from build123d import *

# Parameters (mm, degrees)
SKETCH1_W               = 260
SKETCH1_H               = 60
BOSS_EXTRUDE1_DEPTH     = 5
SKETCH2_W               = 5
SKETCH2_H               = 30
SKETCH2_W_2             = 220
SKETCH2_H_2             = 3
CUT_EXTRUDE1_DEPTH      = 140.73546436
CUT_EXTRUDE2_DEPTH      = 140.73546436
CUT_EXTRUDE2_DEPTH_BACK = 140.73546436
SKETCH3_R               = 1.45
SKETCH3_R_2             = 1.95


with BuildPart() as part:
    # Sketch1 → Boss-Extrude1 (new body)
    with BuildSketch(Plane.XY):
        with Locations((0, 21)):
            Rectangle(SKETCH1_W, SKETCH1_H)
    extrude(amount=BOSS_EXTRUDE1_DEPTH)

    # Sketch2 → Cut-Extrude1 (cut, through all)
    with BuildSketch(Plane.XY.offset(5)):
        with Locations((-127.5, 21)):
            Rectangle(SKETCH2_W, SKETCH2_H)
        with Locations((0, 49.5)):
            Rectangle(SKETCH2_W_2, SKETCH2_H_2)
        with Locations((127.5, 21)):
            Rectangle(SKETCH2_W, SKETCH2_H)
        with BuildLine():
            Line((108, -2), (-108, -2))
            ThreePointArc((-108, -2), (-103.050252532, -4.050252532), (-101, -9))
            Line((-101, -9), (101, -9))
            ThreePointArc((101, -9), (103.050252532, -4.050252532), (108, -2))
        make_face()
        with BuildLine():
            Line((108, -9), (115, -9))
            ThreePointArc((115, -9), (112.949747468, -4.050252532), (108, -2))
            Line((108, -2), (108, -9))
        make_face()
        with BuildLine():
            Line((108, -9), (108, -2))
            ThreePointArc((108, -2), (103.050252532, -4.050252532), (101, -9))
            Line((101, -9), (108, -9))
        make_face()
        with BuildLine():
            ThreePointArc((-108, -2), (-112.949747468, -4.050252532), (-115, -9))
            Line((-115, -9), (-108, -9))
            Line((-108, -9), (-108, -2))
        make_face()
        with BuildLine():
            ThreePointArc((-101, -9), (-103.050252532, -4.050252532), (-108, -2))
            Line((-108, -2), (-108, -9))
            Line((-108, -9), (-101, -9))
        make_face()
    extrude(amount=-CUT_EXTRUDE1_DEPTH, mode=Mode.SUBTRACT)

    # Sketch3 → Cut-Extrude2 (cut, two sides: drawn at the far end of the back side and taken through both)
    with BuildSketch(Plane.XY.offset(5).offset(-CUT_EXTRUDE2_DEPTH_BACK)):
        Polygon((-96.45, 43.2), (-96.45, 40), (-93.55, 40), (-93.55, 43.2), (-92.325, 43.2), (-92.325, 45.5), (-93.55, 45.5), (-93.55, 48), (-96.45, 48), (-96.45, 45.5), (-97.675, 45.5), (-97.675, 43.2), align=None)
        Polygon((97.675, 43.2), (97.675, 45.5), (96.45, 45.5), (96.45, 48), (93.55, 48), (93.55, 45.5), (92.325, 45.5), (92.325, 43.2), (93.55, 43.2), (93.55, 40), (96.45, 40), (96.45, 43.2), align=None)
        Polygon((125, 21.55), (125, 24.45), (122.5, 24.45), (122.5, 25.675), (120.2, 25.675), (120.2, 24.45), (117, 24.45), (117, 21.55), (120.2, 21.55), (120.2, 20.325), (122.5, 20.325), (122.5, 21.55), align=None)
        Polygon((-2.675, 45.5), (-2.675, 43.2), (-1.45, 43.2), (-1.45, 40), (1.45, 40), (1.45, 43.2), (2.675, 43.2), (2.675, 45.5), (1.45, 45.5), (1.45, 48), (-1.45, 48), (-1.45, 45.5), align=None)
        Polygon((-120.2, 21.55), (-117, 21.55), (-117, 24.45), (-120.2, 24.45), (-120.2, 25.675), (-122.5, 25.675), (-122.5, 24.45), (-125, 24.45), (-125, 21.55), (-122.5, 21.55), (-122.5, 20.325), (-120.2, 20.325), align=None)
        with Locations((-127.5, 43.5)):
            Circle(SKETCH3_R)
        with Locations((-127.5, -3)):
            Circle(SKETCH3_R)
        with Locations((127.5, -3)):
            Circle(SKETCH3_R)
        with Locations((127.5, 43.5)):
            Circle(SKETCH3_R)
        with Locations((-95, 9)):
            Circle(SKETCH3_R_2)
        with Locations((95, 9)):
            Circle(SKETCH3_R_2)
        with Locations((0, 9)):
            Circle(SKETCH3_R_2)
    extrude(amount=CUT_EXTRUDE2_DEPTH + CUT_EXTRUDE2_DEPTH_BACK, mode=Mode.SUBTRACT)


solid = part.part
Design review of the part built by this model. Coordinates are the model's own, in mm. A direction names the side the tool comes from. Give positions to 0.01 mm unless a question says otherwise; leave off trailing zeros. Order: outer loops, then holes, each group sorted by start corner. A loop starts at its lowest first (then second) coordinate and runs counter-clockwise, first axis right, second up. Notation, with made-up numbers: (-39.5, 20) - (-14.5, 20) arc R16 cw to (-14.5, 44) - close; hole circle Ø5 at (-28, 82.5). An arc over 180 degrees is marked (long way). Use CSV: the item, a comma, the result in double quotes. Start each with the question number.
Q1. For line 1 (Y direction, x = -127.5, z = 2.85); line 2 (X direction, y = 43.5, z = 3) (3 decimals); line 3 (X direction, y = 9, z = 2.6), list the stretches that pass through material, from the lowest coordinate up.
Q2. Take a section at A-A (z = 2.9). Count the separate pieces of the cut face and the enclosed holes in it, and give its area (3 significant figures).
Q3. For P1, Ø2.5, axis at x = 104, z = 2.5, coming from the +Y side; P2, Ø2, axis at y = 29.5, z = 1.5, coming from the -X side; P3, Ø1.5, axis at y = 23, z = 3, coming from the +X side; P4, Ø4, axis at x = 103.5, y = 34.5, coming from the -Z side, all flat-tipped, find the tip position at first contact; note any pin that passes through.
Q4. Take a section at C-C (x = -65). State the section outline as (y, z) points.
Q5. Take a section at B-B (y = 29). State the section outline as (x, z) points, and give its area (3 significant figures).
Q6. Draft analysis for pull direction X (two halves, no side actions). For faces 5 (the face through (130, 43, 2)), 6 (the face through (103, 48, 3)), 7 (the face through (-2, 21, 5)), state which applies: pulls with the +X half, pulls with the -X half, needs draft (parallel to the pull), parting line crosses it, or undercut.
Q7. Machinability: for faces 1 (the face through (113, -4.1, 2.5)), 2 (the face through (-103, 48, 3)), 3 (the face through (127, 36, 3)), 4 (the face through (-128, 6, 3)), which of the approach directions +Z, -Z, +X, -X, +Y, -Y give a long, thin tool a straight path to every point of the face, cutting with its end or side? Answer none if there is none.
Calculated:
1,line 1,"y = -9 to -4.45, -1.55 to 6, 36 to 42.05, 44.95 to 51"
1,line 2,"x = -130 to -128.95, -126.05 to -97.675, -92.325 to -2.675, 2.675 to 92.325, 97.675 to 126.05, 128.95 to 130"
1,line 3,"x = -125 to -96.95, -93.05 to -1.95, 1.95 to 93.05, 96.95 to 125"
2,separate pieces,"1"
2,enclosed holes,"7"
2,area,"12,800 mm²"
3,P1,"stops at y = 48"
3,P2,"stops at x = -125"
3,P3,"stops at x = 117"
3,P4,"stops at z = 0"
4,outline,"(-2, 0) - (48, 0) - (48, 5) - (-2, 5) - close"
5,outline,"(-125, 0) - (125, 0) - (125, 5) - (-125, 5) - close"
5,area,"1,250 mm²"
6,face 5,"pulls with the +X half"
6,face 6,"undercut"
6,face 7,"needs draft"
7,face 1,"+Z, -Z, -Y"
7,face 2,"+Z, -Z, +Y"
7,face 3,"+Z, -Z, +X"
7,face 4,"+Z, -Z, -X"
